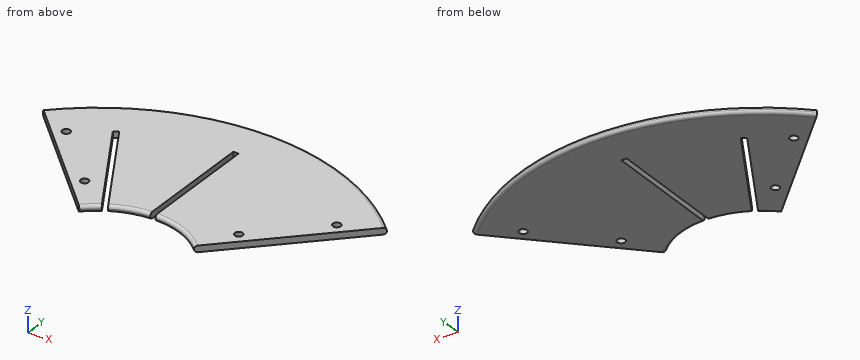
Autodesk Inventor part; units mm, degrees
ref_plane "YZ Plane" through (0, 0, 0) normal (1, 0, 0) x (0, 1, 0)
ref_plane "XZ Plane" through (0, 0, 0) normal (0, 1, 0) x (-1, 0, 0)
ref_plane "XY Plane" through (0, 0, 0) normal (0, 0, 1) x (1, 0, 0)
sketch "Sketch1" plane through (0, 0, 0) normal (0, 0, 1) x (1, 0, 0)
  arc A0 (107.7631, -107.7631) -> (-107.7631, 107.7631) centre (0, 0) ccw
  line L0 (152.4, 0) -> (127, 0)
  line L1 (127, -1.66) -> (127, 1.66)
  line L2 (127, 1.66) -> (50.7729, 1.66)
  line L3 (50.7729, -1.66) -> (127, -1.66)
  line L4 (-64.9376, 109.1552) -> (-26.824, 43.1406)
  line L5 (-23.9488, 44.8006) -> (-62.0624, 110.8152)
  line L6 (-1.66, 127) -> (-1.66, 50.7729)
  line L7 (1.66, 50.7729) -> (1.66, 127)
  line L8 (1.66, 127) -> (-1.66, 127)
  line L9 (-62.0624, 110.8152) -> (-64.9376, 109.1552)
  line L10 (35.921, 35.921) -> (107.7631, 107.7631)
  line L11 (0, 0) -> (152.4, 0) construction
  line L12 (0, 0) -> (152.4, 0) construction
  line L13 (107.7631, -107.7631) -> (35.921, -35.921)
  line L14 (-35.921, 35.921) -> (-107.7631, 107.7631)
  arc A1 (-26.824, 43.1406) -> (-35.921, 35.921) centre (0, 0) ccw
  arc A2 (35.921, -35.921) -> (1.66, 50.7729) centre (0, 0) ccw
  arc A3 (-1.66, 50.7729) -> (-23.9488, 44.8006) centre (0, 0) ccw
  line L15 (35.921, 35.921) -> (53.5987, 53.5987)
  line L16 (107.7631, 107.7631) -> (90.0854, 90.0854)
  circle A4 centre (53.5987, 53.5987) radius 15
  line L17 (53.5987, 53.5987) -> (58.902, 48.2954)
  line L18 (53.5987, 53.5987) -> (48.2954, 58.902)
  circle A5 centre (48.2954, 58.902) radius 2.5
  circle A6 centre (58.902, 48.2954) radius 2.5
  circle A7 centre (90.0854, 90.0854) radius 15
  line L19 (90.0854, 90.0854) -> (95.3887, 84.7821)
  line L20 (90.0854, 90.0854) -> (84.7821, 95.3887)
  circle A8 centre (84.7821, 95.3887) radius 2.5
  circle A9 centre (95.3887, 84.7821) radius 2.5
  line L21 (-90.0854, 90.0854) -> (-84.7821, 95.3887)
  circle A10 centre (-84.7821, 95.3887) radius 2.5
  circle A11 centre (-90.0854, 90.0854) radius 15
  line L22 (-90.0854, 90.0854) -> (-95.3887, 84.7821)
  circle A12 centre (-95.3887, 84.7821) radius 2.5
  circle A13 centre (-58.902, 48.2954) radius 2.5
  circle A14 centre (-53.5987, 53.5987) radius 15
  line L23 (-53.5987, 53.5987) -> (-58.902, 48.2954)
  circle A15 centre (-48.2954, 58.902) radius 2.5
  line L24 (-53.5987, 53.5987) -> (-48.2954, 58.902)
  line L25 (90.0854, -90.0854) -> (84.7821, -95.3887)
  circle A16 centre (84.7821, -95.3887) radius 2.5
  circle A17 centre (90.0854, -90.0854) radius 15
  line L26 (90.0854, -90.0854) -> (95.3887, -84.7821)
  circle A18 centre (95.3887, -84.7821) radius 2.5
  circle A19 centre (58.902, -48.2954) radius 2.5
  circle A20 centre (53.5987, -53.5987) radius 15
  line L27 (53.5987, -53.5987) -> (58.902, -48.2954)
  circle A21 centre (48.2954, -58.902) radius 2.5
  line L28 (53.5987, -53.5987) -> (48.2954, -58.902)
  point P0 (50.8, 0)
  dimension "d2" = 25.4
  dimension "d3" = 3.32
  dimension "d10" = 45
  dimension "d12" = 25
  dimension "d13" = 25
  dimension "d14" = 30
  dimension "d15" = 7.5
  dimension "d16" = 7.5
  dimension "d17" = 5
  dimension "d18" = 5
  dimension "d19" = 30
  dimension "d20" = 7.5
  dimension "d21" = 7.5
  dimension "d22" = 5
  dimension "d23" = 5
extrude "Extrusion2" [suppressed]
extrude "Extrusion3" [suppressed]
extrude "Extrusion4" add sketch "Sketch1" along normal mid plane 4 contours L10 A7 A4 A2 L7 L8 L6 A3 L5 L9 L4 A1 L14 A14 A11 A0 | L10 A7 | A11 L14 | L10 A4 | A14 L14 picked at (92.6865, 95.3887) picked at (-92.6855, 95.3478) picked at (56.1998, 58.902) picked at (-56.1988, 58.8611)
fillet "Fillet1" [suppressed]
fillet "Fillet2" radius 2 6 edges at (-31.5795, 39.7916, 2) (-31.5795, 39.7916, -2) (-13.148, 49.069, 2) (-13.148, 49.069, -2) (20.2046, 46.6091, 2) (20.2046, 46.6091, -2)
fillet "Fillet3" radius 2 2 edges at (0, 152.4, 2) (0, 152.4, -2)
properties part number "fin_alignment_rig_part1"
Geometry: final body of the model. Coordinates: model frame, mm. Give positions to 0.01 mm unless a question says otherwise; leave off trailing zeros. Loops run counter-clockwise (first coordinate to the right, second up) from the corner with the lowest first, then second, coordinate; pieces in that order, holes last. Notation, with made-up numbers: M -17,-22 L 15,-22 A23 ccw 15,12 Z; hole C 40,22.5 d6. An arc over 180 degrees is marked long. Put each result on its own line as item: value.
1) Cut plane C-C, the plane y = 66.5. Return the cut outline in (x, z).
Computed values:
outline: M -66.5,-2 L -40.31,-2 L -40.31,2 L -66.5,2 Z; M -36.48,-2 L -1.66,-2 L -1.66,2 L -36.48,2 Z; M 1.66,-2 L 66.5,-2 L 66.5,2 L 1.66,2 Z
2) First-contact query: P1, Ø3, axis at x = 48.3, y = 58.9, coming from the -Z side; P2, Ø2, axis at y = 100, z = 0.5, coming from the -X side. Flat tips, straight axial feed; report the tip coordinate or a pass-through.
Computed values:
P1: passes through
P2: stops at x = -101
3) Material intervals for L1, parallel to X at y = 78, z = 1.8; L2, parallel to X at y = 63, z = -0.25; L3, parallel to X at y = 114, z = 1.4, sorted ascending. Write a range as from..to.
Computed values:
L1: x = -78..-46.95, -43.12..-1.66, 1.66..78
L2: x = -63..-38.29, -34.46..-1.66, 1.66..63
L3: x = -100.28..-1.66, 1.66..100.28
4) Cut plane B-B, the plane z = -0.85. Return the cut outline in (x, y), plus the area to 3 significant figures.
Computed values:
outline: M -107.63,107.63 L -36.05,36.05 A50.99 cw -26.92,43.3 L -64.94,109.16 L -62.06,110.82 L -24.04,44.96 A50.99 cw -1.66,50.96 L -1.66,127 L 1.66,127 L 1.66,50.96 A50.99 cw 36.05,36.05 L 107.63,107.63 A152.21 ccw Z; hole C -84.78,95.39 d5; hole C -48.3,58.9 d5; hole C 48.3,58.9 d5; hole C 84.78,95.39 d5
area: 15,600 mm^2
5) Cut plane A-A, the plane y = 85.5. Return the cut outline in (x, z), plus the area to 3 significant figures.
Computed values:
outline: M -85.5,-2 L -51.28,-2 L -51.28,2 L -85.5,2 Z; M -47.45,-2 L -1.66,-2 L -1.66,2 L -47.45,2 Z; M 1.66,-2 L 85.5,-2 L 85.5,2 L 1.66,2 Z
area: 655 mm^2
